Design review of the part built by this model. Coordinates are the model's own, in mm. A direction names the side the tool comes from. Coordinates: 2 decimals unless noted, no trailing zeros. Write each loop counter-clockwise with the first axis right and the second up, starting at its lowest first coordinate (ties: lowest second). Pieces come first, ordered by that corner, then holes.
Q1. Take a section at C-C (x = 16). Give the boundary of the cut face in (y, z).
Q2. Take a section at A-A (y = 0). Give the boundary of the cut face in (x, z).
Q3. Machinability: for faces 4 (the flat face through (20.908, -12.046, 33.583)), 5 (the flat face through (-24, 13, 33.02)), 6 (the flat face through (25.192, -12.125, 25.293)), which of the approach directions +Z, -Z, +X, -X, +Y, -Y give a long, thin tool a straight path to every point of the face, cutting with its end or side? Answer none if there is none.
Q4. Insertion check: pin 1 (2 mm diameter, centred on y = 7, z = 18, fed in from +X); pin 2 (10 mm diameter, centred on x = 3, y = -22.5, fed in from +Z); pin 3 (0.9 mm diameter, centred on x = -26, y = -14, fed in from -Z); pin 4 (10 mm diameter, centred on y = 5.5, z = 26, fed in from -X). Each pin has a flat end and moves straight along its axis. Give the tip position at first contact, or say it passes through.
Q5. Take a section at B-B (z = 19). Give the boundary of the cut face in (x, y), and give its area (3 significant figures).
Q6. Mouldability with a two-part tool opening along Z and no side actions: class faces 1 (the flat face through (0, 0, 0)), 2 (the flat face through (-20.89, -12.08, 33.58)), 3 (the flat face through (-22, -13, 33.02)) as pulls with the +Z half, pulls with the -Z half, needs draft (parallel to the pull), parting line crosses it, or undercut.
Q7. Take a section at D-D (z = 15). Give the boundary of the cut face in (x, y).
Q8. For probe 1 along Y at (x, z) = (0, 24); probe 2 along Z at (x, y) = (-20, 5), list the stretches that pass through material, from the lowest coordinate up.
```python
from build123d import *

# Parameters (mm, degrees)
F0_R            = 29.21
F1_DEPTH        = 33.02
F2_R            = 26.67
F3_DEPTH        = 30.48
F4_W            = 3.175
F4_H            = 5.08
F5_DEPTH        = 3.175
F5_COPIES_COUNT = 3
F7_DEPTH        = 3.175
F7_COPIES_COUNT = 3
F8_W            = 0.508
F8_H            = 15.24
F9_DEPTH        = 5.08
F9_COPIES_COUNT = 3


# Not quite as in the source:
# - a pattern or mirror of a feature is missing from the dataset's text; its kind, count and spacing are read off the source's solid


with BuildPart() as f1:
    # F0 (on Top) → F1 (new body)
    with BuildSketch(Plane.XY):
        Circle(F0_R)
    extrude(amount=F1_DEPTH)

    # F2 (on face) → F3 (cut)
    with BuildSketch(Plane.XY.offset(33.02)):
        Circle(F2_R)
    extrude(amount=-F3_DEPTH, mode=Mode.SUBTRACT)

    # F4 (on face) → F5 (join)
    with BuildSketch(Plane.XY.offset(33.02)):
        with Locations((0, 26.67)):
            Rectangle(F4_W, F4_H)
    f5 = extrude(amount=F5_DEPTH)

    # F5_copies: F5 ×3 about axis
    f5_copies_axis = Axis((0, 0, 0), (0, 0, 1))
    for i in range(1, F5_COPIES_COUNT):
        add(f5.rotate(f5_copies_axis, i * 360 / F5_COPIES_COUNT))

    # F6 (on face) → F7 (cut, through all)
    with BuildSketch(Plane(origin=(-1.5875, 0, 0), x_dir=(0, -1, 0), z_dir=(-1, 0, 0))):
        Polygon((-24.13, 36.195), (-27.178, 36.195), (-24.13, 34.163), align=None)
    f7 = extrude(amount=-F7_DEPTH, mode=Mode.SUBTRACT)

    # F7_copies: F7 ×3 about axis
    f7_copies_axis = Axis((0, 0, 0), (0, 0, 1))
    for i in range(1, F7_COPIES_COUNT):
        add(f7.rotate(f7_copies_axis, i * 360 / F7_COPIES_COUNT), mode=Mode.SUBTRACT)

    # F8 (on face) → F9 (cut)
    with BuildSketch(Plane(origin=(0, 29.21, 0), x_dir=(-1, 0, 0), z_dir=(0, 1, 0))):
        with Locations((1.8415, 25.4)):
            Rectangle(F8_W, F8_H)
        with Locations((-1.8415, 25.4)):
            Rectangle(F8_W, F8_H)
    f9 = extrude(amount=-F9_DEPTH, mode=Mode.SUBTRACT)

    # F9_copies: F9 ×3 about axis
    f9_copies_axis = Axis((0, 0, 0), (0, 0, 1))
    for i in range(1, F9_COPIES_COUNT):
        add(f9.rotate(f9_copies_axis, i * 360 / F9_COPIES_COUNT), mode=Mode.SUBTRACT)


solid = f1.part
```
Response:
1. outline: (-24.44, 0) - (24.44, 0) - (24.44, 33.02) - (21.34, 33.02) - (21.34, 2.54) - (-21.34, 2.54) - (-21.34, 33.02) - (-24.44, 33.02) - close
2. outline: (-29.21, 0) - (29.21, 0) - (29.21, 33.02) - (26.67, 33.02) - (26.67, 2.54) - (-26.67, 2.54) - (-26.67, 33.02) - (-29.21, 33.02) - close
3. face 4: +Z, +Y
3. face 5: +Z, -X, +Y
3. face 6: +Z
4. pin 1: stops at x = 28.59
4. pin 2: stops at z = 33.02
4. pin 3: stops at z = 0
4. pin 4: stops at x = -29.21
5. outline: (-26.28, -12.75) - (-24.07, -11.48) arc R26.67 cw to (-2.1, 26.59) - (-2.1, 29.13) arc R29.21 ccw to start; (-26.05, -13.21) arc R29.21 ccw to (-24.47, -15.96) - (-22.26, -14.69) arc R26.67 cw to (-23.85, -11.94) - close; (-24.18, -16.38) arc R29.21 ccw to (24.18, -16.38) - (21.98, -15.11) arc R26.67 cw to (-21.98, -15.11) - close; (-1.59, 26.62) arc R26.67 cw to (1.59, 26.62) - (1.59, 29.17) arc R29.21 ccw to (-1.59, 29.17) - close; (2.1, 26.59) arc R26.67 cw to (24.07, -11.48) - (26.28, -12.75) arc R29.21 ccw to (2.1, 29.13) - close; (22.26, -14.69) - (24.47, -15.96) arc R29.21 ccw to (26.05, -13.21) - (23.85, -11.94) arc R26.67 cw to start
5. area: 438 mm2
6. face 1: pulls with the -Z half
6. face 2: needs draft
6. face 3: undercut
7. outline: circle Ø58.42 at (0, 0); hole circle Ø53.34 at (0, 0)
8. probe 1: y = -29.21 to -26.67, 26.67 to 29.21
8. probe 2: z = 0 to 2.54
